Solid Edge part; units mm, degrees
sketch "Sketch1" plane through (0, 0, 0) normal (0, 0, 1) x (1, 0, 0)
  line L0 (-5.12, 2.07) -> (-5.12, 1.54)
  line L1 (-5.12, 1.54) -> (-4.59, 1.54)
  line L2 (-4.59, 1.54) -> (-4.59, 2.07)
  line L3 (-4.59, 2.07) -> (-5.12, 2.07)
  line L4 (-4.49, 0.13) -> (-4.99, 0.13)
  line L5 (-4.99, 0.13) -> (-4.99, -0.4)
  line L6 (-4.99, -0.4) -> (-4.49, -0.4)
  line L7 (-4.49, -0.4) -> (-4.49, 0.13)
  line L8 (-7.68, -0.26) -> (-6.56, -0.26)
  line L9 (-6.56, -0.26) -> (-6.56, 0.44)
  line L10 (-6.56, 0.44) -> (-7.68, 0.44)
  line L11 (-7.68, 0.44) -> (-7.68, -0.26)
  line L12 (0.44, 0.49) -> (0.44, 4.59)
  line L13 (0.44, 4.59) -> (-6.83, 4.59)
  line L14 (-6.83, 4.59) -> (-6.83, 2.9)
  line L15 (-6.83, 2.9) -> (-8.03, 2.9)
  line L16 (-8.03, 1.18) -> (-8.03, 2.9)
  line L17 (-8.03, 1.18) -> (-8.9351, 1.18)
  line L18 (-8.9351, 1.18) -> (-8.9351, -0.4)
  line L19 (-8.9351, -0.4) -> (-8.03, -0.4)
  line L20 (-8.03, -1.97) -> (-8.03, -0.4)
  line L21 (-8.03, -1.97) -> (-7.23, -1.97)
  line L22 (-7.23, -3.74) -> (-7.23, -1.97)
  line L23 (-7.23, -3.74) -> (0.44, -3.74)
  line L24 (0.44, 0) -> (0.44, -3.74)
  line L25 (0.28, 0) -> (0.44, 0)
  line L26 (0.28, -1.97) -> (0.28, 0)
  line L27 (-2.12, -1.97) -> (0.28, -1.97)
  line L28 (-2.12, 0) -> (-2.12, -1.97)
  line L29 (-2.12, 0) -> (0, 0)
  line L30 (0, 0.49) -> (0, 0)
  line L31 (0.44, 0.49) -> (0, 0.49)
  dimension "D1" = 2.12
  dimension "D2" = 6.56
  dimension "D3" = 6.56
extrude "Protrusion1" add sketch "Sketch1" along normal blind 0.22
sketch "Sketch2" plane through (0.44, -1.78, 0.11) normal (1, 0, 0) x (0, 1, 0)
  line L0 (-0.5536, -0.11) -> (-0.8579, -0.48)
  line L1 (-0.8579, -0.48) -> (-1.96, -0.48)
  line L2 (-1.96, -0.48) -> (-1.96, -0.11)
  line L3 (-0.5536, -0.11) -> (-1.96, -0.11)
extrude "Protrusion2" add sketch "Sketch2" against normal up to surface (7.67 mm away)
sketch "Sketch3" plane through (0.44, -1.78, -0.075) normal (1, 0, 0) x (0, 1, 0)
  line L0 (-1.96, 0.005) -> (-0.7666, 0.005)
  line L1 (-0.528, 0.295) -> (-0.7666, 0.005)
  line L2 (-1.96, 0.295) -> (-0.528, 0.295)
  line L3 (-1.96, 0.005) -> (-1.96, 0.295)
extrude "Cutout1" cut sketch "Sketch3" against normal through all
sketch "Sketch4" plane through (0.44, 2.54, 0.11) normal (1, 0, 0) x (0, 1, 0)
  line L0 (0.7792, -0.36) -> (0.5736, -0.11)
  line L1 (0.5736, -0.11) -> (2.05, -0.11)
  line L2 (2.05, -0.11) -> (2.05, -0.36)
  line L3 (0.7792, -0.36) -> (2.05, -0.36)
  dimension "D1" = 2.05
extrude "Protrusion3" add sketch "Sketch4" against normal up to surface (7.27 mm away)
sketch "Sketch5" plane through (0.44, 2.54, -0.015) normal (1, 0, 0) x (0, 1, 0)
  line L0 (0.548, 0.235) -> (2.05, 0.235)
  line L1 (2.05, 0.235) -> (2.05, 0.065)
  line L2 (2.05, 0.065) -> (0.6878, 0.065)
  line L3 (0.548, 0.235) -> (0.6878, 0.065)
extrude "Cutout2" cut sketch "Sketch5" against normal through all
sketch "Sketch6" plane through (-8.4826, 1.18, 0.11) normal (0, 1, 0) x (-1, 0, 0)
  line L0 (-0.43, -0.56) -> (-0.6468, -0.11)
  line L1 (-0.6468, -0.11) -> (0.4526, -0.11)
  line L2 (0.4526, -0.11) -> (0.4526, -0.56)
  line L3 (-0.43, -0.56) -> (0.4526, -0.56)
  dimension "D1" = 0.4526
extrude "Protrusion4" add sketch "Sketch6" against normal up to surface (1.58 mm away)
sketch "Sketch7" plane through (-8.03, 2.04, 0.11) normal (-1, 0, 0) x (0, -1, 0)
  line L0 (-0.86, 0.11) -> (-0.86, -0.11)
  line L1 (-0.86, -0.11) -> (-1.229, -0.11)
  line L2 (-1.229, -0.11) -> (-1.048, 0.11)
  line L3 (-1.048, 0.11) -> (-0.86, 0.11)
  line L4 (4.01, 0.11) -> (4.01, -0.11)
  line L5 (4.529, -0.11) -> (4.01, -0.11)
  line L6 (4.529, -0.11) -> (4.348, 0.11)
  line L7 (4.01, 0.11) -> (4.348, 0.11)
extrude "Protrusion5" add sketch "Sketch7" against normal up to last
sketch "Sketch8" plane through (-8.4825, 1.18, -0.115) normal (0, 1, 0) x (-1, 0, 0)
  line L0 (-0.6195, 0.335) -> (0.4526, 0.335)
  line L1 (0.4526, 0.335) -> (0.4526, -0.035)
  line L2 (0.4526, -0.035) -> (-0.4413, -0.035)
  line L3 (-0.4413, -0.035) -> (-0.6195, 0.335)
extrude "Cutout3" cut sketch "Sketch8" along normal through all and the other way through all
sketch "Sketch9" plane through (0.28, -1.05, 0.11) normal (-1, 0, 0) x (0, 1, 0)
  line L0 (-0.92, -0.11) -> (-0.92, 0.11)
  line L1 (-0.92, 0.11) -> (-1.2836, 0.11)
  line L2 (-1.2836, 0.11) -> (-1.1026, -0.11)
  line L3 (-0.92, -0.11) -> (-1.1026, -0.11)
extrude "Cutout4" cut sketch "Sketch9" along normal up to surface (2.4 mm away)
sketch "Sketch10" plane through (0.44, 2.54, -0.015) normal (1, 0, 0) x (0, 1, 0)
  line L0 (2.05, 0.065) -> (2.05, -0.235)
  line L1 (2.05, -0.235) -> (0.9346, -0.235)
  line L2 (0.6878, 0.065) -> (0.9346, -0.235)
  line L3 (2.05, 0.065) -> (0.6878, 0.065)
  line L4 (-6.28, -0.355) -> (-5.3333, -0.355)
  line L5 (-5.0866, -0.055) -> (-5.3333, -0.355)
  line L6 (-6.28, -0.055) -> (-5.0866, -0.055)
  line L7 (-6.28, -0.055) -> (-6.28, -0.355)
extrude "Ausschnitt_7" cut sketch "Sketch10" against normal blind 0.001
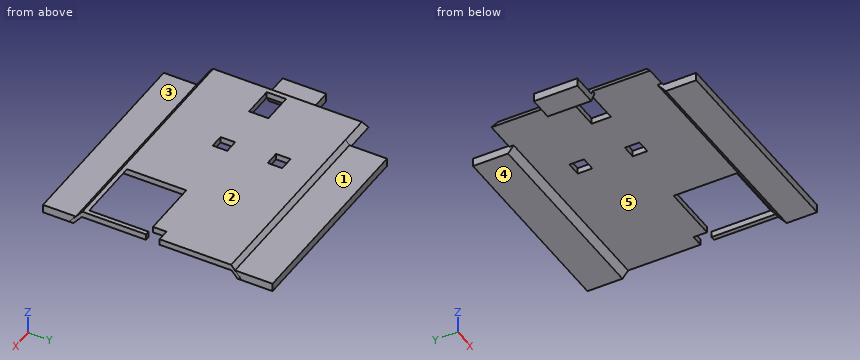
The model under review builds one solid part; all positions refer to its coordinate system, in mm. Face numbers are marked on the shaded views. A direction names the side the tool comes from. Give positions to 0.01 mm unless a question says otherwise; leave off trailing zeros. Order: outer loops, then holes, each group sorted by start corner. A loop starts at its lowest first (then second) coordinate and runs counter-clockwise, first axis right, second up. Notation, with made-up numbers: (77, -26.75) - (128, -26.75) arc R23 cw to (128, -8.75) - close; hole circle Ø11 at (46, 21.5). An arc over 180 degrees is marked (long way). Use CSV: the item, a comma, the result in double quotes. Start each with the question number.
Q1. We need section D-D, the plane x = -5.25. Write out the cut boundary in (y, z), and give its area (3 significant figures).
Q2. Clearance check with flat-ended pins moving along their axes: pin 1 Ø4 at (x, y) = (-1, 1) entering from -Z; pin 2 Ø4 at (x, y) = (-6.5, 0.5) entering from -Z. State where each tip first meets the part, or that it passes through.
Q3. Tool access review of the marked faces 1, 2 and 3: name each direction out of +Z, -Z, +X, -X, +Y, -Y from which nothing blocks a thin tool from reaching the whole face with its end or side.
Q4. We need section A-A, the plane x = -1.75. Write out the cut boundary in (y, z).
Q5. We need section C-C, the plane x = -7. Write out the cut boundary in (y, z), and give its area (3 significant figures).
Q6. The part is to be moulded in two halves that separate along Y. For the marked faces 4 and 5, say which applies: +Y half, -Y half, draft (parallel to the pull), parting line (faces both ways), or undercut.
Q7. To check wall thickness, follow line 1 along X through (y, z) = (3.75, -0.05); line 2 along Z through (x, y) = (-5.75, 0); line 3 along Y through (x, z) = (-1, -0.2). State the ranges of each line that lie inside material, in increasing order. Write a range as [from, to].
Q8. We need section B-B, the plane y = -2. Write out the cut boundary in (x, z), and give its area (3 significant figures).
Outcome:
1,outline,"(-3.74, -0.37) - (-2.64, -0.37) - (-2.33, 0) - (3.11, 0) - (3.32, -0.25) - (4.59, -0.25) - (4.59, 0.05) - (3.23, 0.05) - (3.09, 0.22) - (-2.31, 0.22) - (-2.55, -0.07) - (-3.74, -0.07) - close"
1,area,"2.02 mm^2"
2,pin 1,"stops at z = 0"
2,pin 2,"stops at z = -0.45"
3,face 1,"+Z, +X, -X, +Y"
3,face 2,"+Z, +X, -X, +Y, -Y"
3,face 3,"+Z, +X, -X, -Y"
4,outline,"(-3.74, -0.37) - (-2.64, -0.37) - (-2.33, 0) - (-2.15, 0.22) - (-2.31, 0.22) - (-2.55, -0.07) - (-3.74, -0.07) - close; (0, 0) - (3.11, 0) - (3.32, -0.25) - (4.59, -0.25) - (4.59, 0.05) - (3.23, 0.05) - (3.09, 0.22) - (0, 0.22) - close"
5,outline,"(-3.74, -0.37) - (-2.64, -0.37) - (-2.33, 0) - (-0.26, 0) - (-0.26, 0.22) - (-2.31, 0.22) - (-2.55, -0.07) - (-3.74, -0.07) - close; (0.44, 0) - (3.27, 0) - (3.09, 0.22) - (0.44, 0.22) - close"
5,area,"1.45 mm^2"
6,face 4,"draft"
6,face 5,"undercut"
7,line 1,"x = [-6.83, 0.44]"
7,line 2,"z = [0, 0.22]"
7,line 3,"y = [-3.74, -2.5], [3.28, 4.59]"
8,outline,"(-7.97, 0) - (-2.12, 0) - (-2.12, 0.22) - (-7.86, 0.22) - close; (0.28, 0) - (0.44, 0) - (0.44, 0.22) - (0.28, 0.22) - close"
8,area,"1.31 mm^2"
